```python
from build123d import *

# Parameters (mm, degrees)
SKETCH1_W           = 254
SKETCH1_H           = 6.35
BOSS_EXTRUDE1_DEPTH = 304.8
CUT_EXTRUDE1_DEPTH  = 304.8
CUT_EXTRUDE2_DEPTH  = 397.811494919
CUT_EXTRUDE3_REACH  = 398.811
FILLET2_R           = 2.54


with BuildPart() as part:
    # Sketch1 → Boss-Extrude1 (new body)
    with BuildSketch(Plane.XY):
        with Locations((-127, 3.175)):
            Rectangle(SKETCH1_W, SKETCH1_H)
    extrude(amount=BOSS_EXTRUDE1_DEPTH)

    # Sketch2 → Cut-Extrude1 (cut)
    with BuildSketch(Plane(origin=(0, 6.35, 0), x_dir=(1, 0, 0), z_dir=(0, 1, 0))):
        Polygon((-101.6, -304.8), (-254, 0), (-254, -304.8), align=None)
    extrude(amount=-CUT_EXTRUDE1_DEPTH, mode=Mode.SUBTRACT)

    # Sketch4 → Cut-Extrude2 (cut, through all)
    with BuildSketch(Plane(origin=(0, 6.35, 0), x_dir=(1, 0, 0), z_dir=(0, 1, 0))):
        Polygon((-76.2, -127), (-76.2, 0), (0, 0), (0, -304.8), (-76.2, -304.8), (-76.2, -177.8), align=None)
    extrude(amount=-CUT_EXTRUDE2_DEPTH, mode=Mode.SUBTRACT)

    # Sketch9 → Cut-Extrude3 (cut, up to next)
    with BuildSketch(Plane(origin=(0, 6.35, 0), x_dir=(1, 0, 0), z_dir=(0, 1, 0)), mode=Mode.PRIVATE) as cut_extrude3_sk1:
        with BuildLine():
            Line((-102.249215459, -33.393768297), (-167.865313489, -127.103267909))
            ThreePointArc((-167.865313489, -127.103267909), (-172.400201066, -129.255743451), (-176.570296004, -126.461344677))
            Line((-176.570296004, -126.461344677), (-223.42504581, -32.751845065))
            ThreePointArc((-223.42504581, -32.751845065), (-223.202661786, -27.80928595), (-218.88135568, -25.4))
            Line((-218.88135568, -25.4), (-106.410507844, -25.4))
            ThreePointArc((-106.410507844, -25.4), (-101.904492811, -28.134317045), (-102.249215459, -33.393768297))
        make_face()
    cut_extrude3_tool1 = extrude(cut_extrude3_sk1.sketch, amount=-CUT_EXTRUDE3_REACH, mode=Mode.PRIVATE) & part.part
    # Sketch9 → Cut-Extrude3 (cut, up to next)
    with BuildSketch(Plane(origin=(0, 6.35, 0), x_dir=(1, 0, 0), z_dir=(0, 1, 0)), mode=Mode.PRIVATE) as cut_extrude3_sk2:
        with BuildLine():
            Line((-158.13257617, -146.897559021), (-93.98, -146.897559021))
            ThreePointArc((-93.98, -146.897559021), (-90.387897552, -148.385456572), (-88.9, -151.977559021))
            Line((-88.9, -151.977559021), (-88.9, -280.28271136))
            ThreePointArc((-88.9, -280.28271136), (-92.812855164, -285.226816227), (-98.52369013, -282.554556425))
            Line((-98.52369013, -282.554556425), (-162.6762663, -154.249404086))
            ThreePointArc((-162.6762663, -154.249404086), (-162.453882276, -149.306844971), (-158.13257617, -146.897559021))
        make_face()
    cut_extrude3_tool2 = extrude(cut_extrude3_sk2.sketch, amount=-CUT_EXTRUDE3_REACH, mode=Mode.PRIVATE) & part.part
    # Sketch9 → Cut-Extrude3 (cut, up to next)
    with BuildSketch(Plane(origin=(0, 6.35, 0), x_dir=(1, 0, 0), z_dir=(0, 1, 0)), mode=Mode.PRIVATE) as cut_extrude3_sk3:
        with BuildLine():
            Line((-98.141292385, -49.668820452), (-151.731655506, -126.203790724))
            ThreePointArc((-151.731655506, -126.203790724), (-152.076378154, -131.463241976), (-147.570363121, -134.197559021))
            Line((-147.570363121, -134.197559021), (-93.98, -134.197559021))
            ThreePointArc((-93.98, -134.197559021), (-90.387897552, -132.709661469), (-88.9, -129.117559021))
            Line((-88.9, -129.117559021), (-88.9, -52.582588748))
            ThreePointArc((-88.9, -52.582588748), (-92.452414539, -47.737706638), (-98.141292385, -49.668820452))
        make_face()
    cut_extrude3_tool3 = extrude(cut_extrude3_sk3.sketch, amount=-CUT_EXTRUDE3_REACH, mode=Mode.PRIVATE) & part.part
    add(cut_extrude3_tool1.solids().sort_by_distance((-165.555188, 6.35, 61.646702))[0], mode=Mode.SUBTRACT)
    add(cut_extrude3_tool2.solids().sort_by_distance((-114.904844, 6.35, 197.54946))[0], mode=Mode.SUBTRACT)
    add(cut_extrude3_tool3.solids().sort_by_distance((-111.777944, 6.35, 102.228886))[0], mode=Mode.SUBTRACT)

    # Fillet2
    fillet2_edges = [part.edges().sort_by_distance(p)[0] for p in [
        (-177.8, 0, 152.4),
        (-177.8, 6.35, 152.4),
        (-101.6, 3.175, 304.8),
        (-165.1, 0, 0),
        (-165.1, 6.35, 0),
        (-88.9, 6.35, 304.8),
        (-88.9, 0, 304.8),
        (-76.2, 6.35, 152.4),
        (-76.2, 3.175, 304.8),
        (-76.2, 3.175, 0),
        (-76.2, 0, 152.4),
        (-254, 3.175, 0),
    ]]
    fillet(fillet2_edges, radius=FILLET2_R)


solid = part.part
```
Check sheet for the modelled part. Datum: model origin and axes. Units: mm. A direction names the side the tool comes from. Coordinates: 2 decimals unless noted, no trailing zeros. Write each loop counter-clockwise with the first axis right and the second up, starting at its lowest first coordinate (ties: lowest second). Pieces come first, ordered by that corner, then holes. Notation, with made-up numbers: M 50.5,-8.5 L 98.5,-8.5 A29 ccw 98.5,22.5 Z; hole C -21.75,58 d10. An arc over 180 degrees is marked long. Use one line per item in the form item = value.
Item 1: Release check for a two-part mould opening along X. For faces 3 (the face through (-130.15, 3.22, 219.3)), 4 (the face through (-146, 0, 107)), 5 (the face through (-177.63, 0.76, 151.11)) record: pulls with the +X half, pulls with the -X half, needs draft (parallel to the pull), parting line crosses it, or undercut.
Answer below:
face_3 = undercut
face_4 = needs draft
face_5 = pulls with the -X half
Item 2: Material ranges on L1, parallel to Z at x = -115.5, y = 2.5; L2, parallel to Z at x = -103, y = 5; L3, parallel to Z at x = -199.5, y = 4, recorded low to high. Write a range as from..to.
Answer below:
L1 = 0..25.4, 52.32..74.46, 134.2..146.9, 248.6..277
L2 = 0.3..26.72, 34.47..56.61, 134.2..146.9, 273.6..301.34
L3 = 0.01..25.4, 80.6..108.98
Item 3: Sectioned sample at B-B, the plane x = -119.5. State how many separate pieces and enclosed holes the cut face has, and give its area (3 significant figures).
Answer below:
separate_pieces = 4
enclosed_holes = 0
area = 554 mm^2
Item 4: Set-up check for faces 1 (the face through (-177.63, 5.59, 151.11)), 2 (the face through (-162.49, 3.22, 149.37)): record each of +Z, -Z, +X, -X, +Y, -Y from which the full face is reachable in a straight line by a thin tool's end or side.
Answer below:
face_1 = +Z, -X, +Y
face_2 = +Y, -Y
Item 5: Gauge pin test, flat ends, axial feed: pin 1 Ø1.9 at (y, z) = (3.5, 218.5) entering from -X (3 decimals); pin 2 Ø1.9 at (x, y) = (-122.5, 4.5) entering from -Z; pin 3 Ø1.9 at (x, y) = (-169, 3) entering from +Z; pin 4 Ø1.5 at (x, y) = (-115.5, 1.5) entering from +Z. Record the tip position at first contact, or that the pin passes through.
Answer below:
pin_1 = -145.225
pin_2 = 0
pin_3 = 171.9
pin_4 = 278.13
Item 6: Sectioned sample at A-A, the plane y = 5.25. Record the cut outline in (x, z).
Answer below:
outline = M -251.76,3.48 A2.09 ccw -249.89,0.45 L -78.74,0.45 A2.09 ccw -76.65,2.54 L -76.65,302.26 A2.09 ccw -78.74,304.35 L -100.03,304.35 A2.09 ccw -101.9,303.2 Z; hole M -223.43,32.75 A5.08 ccw -218.88,25.4 L -106.41,25.4 A5.08 ccw -102.25,33.39 L -167.87,127.1 A5.08 ccw -176.57,126.46 Z; hole M -162.68,154.25 A5.08 ccw -158.13,146.9 L -93.98,146.9 A5.08 ccw -88.9,151.98 L -88.9,280.28 A5.08 ccw -98.52,282.55 Z; hole M -151.73,126.2 L -98.14,49.67 A5.08 ccw -88.9,52.58 L -88.9,129.12 A5.08 ccw -93.98,134.2 L -147.57,134.2 A5.08 ccw Z
